Work out the finished part from the listing and answer in its coordinate system (mm). A direction names the side the tool comes from. Give positions to 0.01 mm unless a question says otherwise; leave off trailing zeros. Order: outer loops, then holes, each group sorted by start corner. A loop starts at its lowest first (then second) coordinate and runs counter-clockwise, first axis right, second up. Notation, with made-up numbers: M 73.5,39.25 L 104.5,39.25 A33 ccw 104.5,75.25 Z; hole C -7,53.5 d10. An arc over 180 degrees is marked long. One line per item, written item: value.
from build123d import *

# Parameters (mm, degrees)
SALIENTE_EXTRUIR1_DEPTH = 58.05
REDONDEO1_R             = 20
REDONDEO2_R             = 20
REDONDEO3_R             = 17
REDONDEO4_R             = 17
CAVIDAD1_START          = -47
CAVIDAD1_DEPTH          = 50
CROQUIS8_W              = 10
CROQUIS8_H              = 3
SALIENTE_EXTRUIR2_DEPTH = 50
CROQUIS9_R              = 2.25
CORTAR_EXTRUIR6_DEPTH   = 136.665712106
SALIENTE_EXTRUIR3_REACH = 146.947
CROQUIS11_W             = 20
CROQUIS11_H             = 3
CROQUIS12_W             = 69.238292886
CROQUIS12_H             = 3
CORTAR_EXTRUIR7_DEPTH   = 1
CROQUIS15_R             = 1.75
CORTAR_EXTRUIR10_DEPTH  = 5
REDONDEO5_R             = 7
REDONDEO6_R             = 3
CROQUIS16_R             = 67.5
CORTAR_EXTRUIR11_DEPTH  = 145.946782753
CROQUIS18_R             = 11
CORTAR_EXTRUIR12_DEPTH  = 146.081609054


# Read off the part's stored shape, not the designer's step: Cavidad1
with BuildPart() as part:
    # Croquis1 → Saliente-Extruir1 (new, symmetric)
    with BuildSketch(Plane(origin=(0, 0, 0), x_dir=(0, 0, -1), z_dir=(1, 0, 0))):
        Polygon((0, 0), (0, 67.196152423), (28.732050808, 116.961524227), (47, 116.961524227), (47, 119.961524227), (27, 119.961524227), (-3, 68), (-3, 0), align=None)
    extrude(amount=SALIENTE_EXTRUIR1_DEPTH, both=True)

    # Redondeo1
    redondeo1_edges = [part.edges().sort_by_distance(p)[0] for p in [
        (0, 68, 3),
    ]]
    fillet(redondeo1_edges, radius=REDONDEO1_R)

    # Redondeo2
    redondeo2_edges = [part.edges().sort_by_distance(p)[0] for p in [
        (0, 119.961524227, -27),
    ]]
    fillet(redondeo2_edges, radius=REDONDEO2_R)

    # Redondeo3
    redondeo3_edges = [part.edges().sort_by_distance(p)[0] for p in [
        (0, 116.961524227, -28.732050808),
    ]]
    fillet(redondeo3_edges, radius=REDONDEO3_R)

    # Redondeo4
    redondeo4_edges = [part.edges().sort_by_distance(p)[0] for p in [
        (0, 67.196152423, 0),
    ]]
    fillet(redondeo4_edges, radius=REDONDEO4_R)

    # Cavidad1 outline → Cavidad1 (cut)
    with BuildSketch(Plane.XY.offset(CAVIDAD1_START)):
        with BuildLine():
            Line((58.05, 0), (58.05, 119.961524227))
            Line((58.05, 119.961524227), (-5.55, 119.961524227))
            Line((-5.55, 119.961524227), (-5.55, 116.961524227))
            Line((-5.55, 116.961524227), (5.123846837, 116.961524227))
            ThreePointArc((5.123846837, 116.961524227), (12.308357287, 115.368756607), (18.14660237, 110.888913592))
            Line((18.14660237, 110.888913592), (51.073651347, 71.647984679))
            ThreePointArc((51.073651347, 71.647984679), (54.025670368, 66.534937751), (55.050895814, 60.720595315))
            Line((55.050895814, 60.720595315), (55.050895814, 0))
            Line((55.050895814, 0), (58.05, 0))
        make_face()
    extrude(amount=CAVIDAD1_DEPTH, mode=Mode.SUBTRACT)

    # Croquis8 → Saliente-Extruir2 (add)
    with BuildSketch(Plane(origin=(0, 0, 0), x_dir=(-1, 0, 0), z_dir=(0, 0, -1))):
        with Locations((-49.050895814, 6.5)):
            Rectangle(CROQUIS8_W, CROQUIS8_H)
    extrude(amount=SALIENTE_EXTRUIR2_DEPTH)

    # Croquis9 → Cortar-Extruir6 (cut, through all)
    with BuildSketch(Plane(origin=(0, 8, 0), x_dir=(1, 0, 0), z_dir=(0, 1, 0))):
        with Locations(Location((49.050895814, 45, 0), (0, 0, 180))):
            Circle(CROQUIS9_R)
    extrude(amount=-CORTAR_EXTRUIR6_DEPTH, mode=Mode.SUBTRACT)

    # Saliente-Extruir3: up to this plane
    saliente_extruir3_end = Plane(origin=(58.05, 67.196152423, 0), z_dir=(0, 0.49999999999999767, 0.86602540378444))
    # Croquis11 → Saliente-Extruir3 (add, up to the surface)
    with BuildSketch(Plane(origin=(0, 0, -54), x_dir=(-1, 0, 0), z_dir=(0, 0, -1)), mode=Mode.PRIVATE) as saliente_extruir3_sk1:
        with Locations((28.05, 92.461524227)):
            Rectangle(CROQUIS11_W, CROQUIS11_H)
    saliente_extruir3_tool1 = split(extrude(saliente_extruir3_sk1.sketch, amount=-SALIENTE_EXTRUIR3_REACH, mode=Mode.PRIVATE), bisect_by=saliente_extruir3_end, keep=Keep.BOTH, mode=Mode.PRIVATE)
    add(saliente_extruir3_tool1.solids().sort_by_distance((-28.05, 92.461524, -54))[0])

    # Croquis12 → Cortar-Extruir7 (cut)
    with BuildSketch(Plane.XZ):
        with Locations((20.431749371, 1.5)):
            Rectangle(CROQUIS12_W, CROQUIS12_H)
    extrude(amount=-CORTAR_EXTRUIR7_DEPTH, mode=Mode.SUBTRACT)

    # Croquis15 → Cortar-Extruir10 (cut)
    with BuildSketch(Plane.XZ.offset(-90.961524227)):
        with Locations(Location((-28.049104186, -49.5, 0), (0, 0, 270))):
            Circle(CROQUIS15_R)
    extrude(amount=-CORTAR_EXTRUIR10_DEPTH, mode=Mode.SUBTRACT)

    # Redondeo5
    redondeo5_edges = [part.edges().sort_by_distance(p)[0] for p in [
        (-18.05, 92.461524227, -54),
        (-38.05, 92.461524227, -54),
    ]]
    fillet(redondeo5_edges, radius=REDONDEO5_R)

    # Redondeo6
    redondeo6_edges = [part.edges().sort_by_distance(p)[0] for p in [
        (54.050895814, 6.5, -50),
        (44.050895814, 6.5, -50),
    ]]
    fillet(redondeo6_edges, radius=REDONDEO6_R)

    # Croquis16 → Cortar-Extruir11 (cut, through all)
    with BuildSketch(Plane.XY.offset(3)):
        with Locations((-45.071920691, 22.721524227)):
            Circle(CROQUIS16_R)
    extrude(amount=-CORTAR_EXTRUIR11_DEPTH, mode=Mode.SUBTRACT)

    # Croquis18 → Cortar-Extruir12 (cut, through all)
    with BuildSketch(Plane(origin=(0, 18.299038106, 31.694863729), x_dir=(1, 0, 0), z_dir=(0, 0.4999999999999976, 0.86602540378444))):
        with Locations(Location((12.350895814, 79.099876042, 0), (0, 0, 270))):
            Circle(CROQUIS18_R)
    extrude(amount=-CORTAR_EXTRUIR12_DEPTH, mode=Mode.SUBTRACT)


solid = part.part
(1) Determine the mould class of faces 3 (the flat face through (44.051, 6, -23)), 4 (the flat face through (-28, 90.962, -34)), 5 (the cylindrical face through (28.821, 67.101, -0.595)), 6 (the cylindrical face through (10.68, 116.03, -30.29)) for opening direction Y: pulls with the +Y half, pulls with the -Y half, needs draft (parallel to the pull), parting line crosses it, or undercut.
Findings:
face 3: needs draft
face 4: pulls with the -Y half
face 5: undercut
face 6: pulls with the +Y half
(2) Section D-D, the plane x = 29 is taken. Give the vertices of the cut face in (y, z).
Findings:
outline: M 1,0 L 62.64,0 A17 cw 71.14,-2.28 L 97.95,-17.76 L 97.95,-14.29 L 72.64,0.32 A20 ccw 62.64,3 L 1,3 Z
(3) Find the intervals of material crossed by probe 1 along Y at (x, z) = (-34.5, -31); probe 2 along X at (y, z) = (92.65, -49.5); probe 3 along Z at (x, y) = (37, 39), in increasing order. Write a range as from..to.
Findings:
probe 1: y = 90.96..93.96, 115.19..118.48
probe 2: x = -37.59..-29.8, -26.3..-18.51
probe 3: z = 0..3
(4) Section B-B, the plane x = 16.5 is taken. Give the vertices of the cut face in (y, z), then the cut area to 3 significant figures.
Findings:
outline: M 50.38,0 L 62.64,0 A17 cw 71.14,-2.28 L 76.48,-5.36 L 77.98,-2.76 L 72.64,0.32 A20 ccw 62.64,3 L 50.38,3 Z; M 94.12,-15.55 L 108.46,-23.82 A17 cw 112.59,-27.17 L 112.59,-23.04 A20 ccw 109.96,-21.23 L 95.62,-12.95 Z
area: 147 mm^2
(5) Which of the six approach directions +Z, -Z, +X, -X, +Y, -Y give full straight-line access (tool end or side, diameter ignored) to faces 1 (the flat face through (49, 5, -25)), 2 (the cylindrical face through (27.27, 67.747, 2.337))?
Findings:
face 1: -Z, +X, -X, -Y
face 2: +Z, +X, -X, +Y
(6) Given P1, Ø8, axis at x = 50.5, z = -22, coming from the +Y side; P2, Ø0.9, axis at y = 7, z = -14.5, coming from the -X side; P3, Ø0.9, axis at x = 49, y = 7, coming from the -Z side, each flat-ended and moving along its own axis, determine where each tip first touches the part or whether it passes through.
Findings:
P1: stops at y = 8
P2: stops at x = 44.05
P3: stops at z = -50
(7) Section C-C, the plane z = -33.5 is taken. Give the vertices of the cut face in (x, y).
Findings:
outline: M -58.05,116.2 L 10.17,116.2 A17 ccw 5.12,116.96 L -5.55,116.96 L -5.55,119.31 L -58.05,119.31 Z; M -38.05,90.96 L -18.05,90.96 L -18.05,93.96 L -38.05,93.96 Z; M 44.05,5 L 54.05,5 L 54.05,8 L 44.05,8 Z
(8) Section A-A, the plane z = -45 is taken. Give the vertices of the cut face in (x, y), then the cut area to 3 significant figures.
Findings:
outline: M -58.05,116.96 L -5.55,116.96 L -5.55,119.96 L -58.05,119.96 Z; M -38.05,90.96 L -18.05,90.96 L -18.05,93.96 L -38.05,93.96 Z; M 44.05,5 L 46.8,5 L 46.8,8 L 44.05,8 Z; M 51.3,5 L 54.05,5 L 54.05,8 L 51.3,8 Z
area: 234 mm^2
